Check sheet for the modelled part. Datum: model origin and axes. Units: mm. A direction names the side the tool comes from. Give positions to 0.01 mm unless a question says otherwise; leave off trailing zeros. Loops run counter-clockwise (first coordinate to the right, second up) from the corner with the lowest first, then second, coordinate; pieces in that order, holes last. Notation, with made-up numbers: (-7.75, 86) -> (20.25, 86) arc R11 cw to (20.25, 95) -> close; hole circle Ø8 at (72.25, 88.5). An arc over 180 degrees is marked (long way). Answer as CSV lines item,"result". Start each with the question number.
(1) Material ranges on line 1 (X direction, y = 23.4, z = 125); line 2 (Z direction, x = 0, y = 195); line 3 (X direction, y = 9, z = -62), recorded low to high. Write a range as from..to.
(2) Gauge pin test, flat ends, axial feed: pin 1 Ø19 at (x, y) = (0, 145) entering from -Z; pin 2 Ø13.5 at (y, z) = (108, 73) entering from -X; pin 3 Ø4 at (y, z) = (22, 116) entering from +X. Record the tip position at first contact, or that the pin passes through.
(3) Access from +Z, -Z, +X, -X, +Y, -Y to the whole of each face (thin tool, end or side, straight path). Record for faces 1 (the face through (-1.301, 150.857, 49.223)), 2 (the face through (-17.5, 131, 75)), 3 (the face through (97, 25, -56)), 4 (the face through (92.07, 22.46, -67.59)), 5 (the face through (106, 16.4, -45)).
(4) Release check for a two-part mould opening along Y. For faces 6 (the face through (-97, 25, -56)), 7 (the face through (2.956, 150.684, 73.907)), 8 (the face through (-47.69, 197.54, -15.02)) record: pulls with the +Y half, pulls with the -Y half, needs draft (parallel to the pull), parting line crosses it, or undercut.
(5) Section check A-A on z = 0. Enter the section's corners in (x, y), plus the area to 3 significant figures.
(6) Section check C-C on x = 0. State how many separate pieces and enclosed holes the cut face has, plus the area to 3 significant figures.
(7) Section check B-B on y = 97. Enter the section's corners in (x, z), plus the area to 3 significant figures.
from build123d import *

# Parameters (mm, degrees)
BOSS_EXTRUDE1_DEPTH = 80
HOLE1_D             = 50
HOLE1_CBORE_D       = 70
HOLE1_CBORE_DEPTH   = 12
BOSS_EXTRUDE2_DEPTH = 10
CIRPATTERN1_COUNT   = 3
FILLET1_R           = 5
HOLE2_D             = 13
HOLE2_CBORE_D       = 22
HOLE2_CBORE_DEPTH   = 5


with BuildPart() as part:
    # Sketch1 → Revolve1 (revolve)
    with BuildSketch(Plane.XY):
        Polygon((-150, 0), (-150, 15), (-106.265538433, 15), (-50, 195), (-50, 200), (0, 200), (0, 0), align=None)
    revolve(axis=Axis((0, 200, 0), (0, -1, 0)))

    # Sketch2 → Boss-Extrude1 (add)
    with BuildSketch(Plane.XY):
        with BuildLine():
            Line((-17.5, 145), (-17.5, 90))
            Line((-17.5, 90), (17.5, 90))
            Line((17.5, 90), (17.5, 145))
            ThreePointArc((17.5, 145), (0, 162.5), (-17.5, 145))
        make_face()
    extrude(amount=BOSS_EXTRUDE1_DEPTH)

    # Sketch4 → Cut-Revolve1 (revolve, cut)
    with BuildSketch(Plane(origin=(0, 0, 0), x_dir=(0, 0, -1), z_dir=(1, 0, 0)), mode=Mode.PRIVATE) as cut_revolve1_sk:
        Polygon((0, 151), (-73.5, 151), (-80, 157.5), (-80, 145), (0, 145), align=None)
    revolve(cut_revolve1_sk.sketch.rotate(Axis((0, 145, 80), (0, 0, -1)), 90), axis=Axis((0, 145, 80), (0, 0, -1)), mode=Mode.SUBTRACT)

    # Hole1 (through all)
    with Locations(Plane(origin=(0, 200, 0), x_dir=(1, 0, 0), z_dir=(0, 1, 0))):
        with Locations((0, 0)):
            CounterBoreHole(HOLE1_D / 2, HOLE1_CBORE_D / 2, HOLE1_CBORE_DEPTH)

    # Sketch7 → Cut-Revolve2 (revolve, cut)
    with BuildSketch(Plane(origin=(0, 0, 0), x_dir=(0, 0, -1), z_dir=(1, 0, 0)), mode=Mode.PRIVATE) as cut_revolve2_sk:
        with BuildLine():
            Line((0, 0), (90, 0))
            Line((90, 0), (53.93166414, 115.38680044))
            ThreePointArc((53.93166414, 115.38680044), (46.296011996, 121), (38.660359853, 115.38680044))
            Line((38.660359853, 115.38680044), (26.973757314, 78))
            Line((26.973757314, 78), (0, 78))
            Line((0, 78), (0, 0))
        make_face()
    revolve(cut_revolve2_sk.sketch.rotate(Axis((0, 78, 0), (0, -1, 0)), 180), axis=Axis((0, 78, 0), (0, -1, 0)), mode=Mode.SUBTRACT)

    # Sketch10 → Boss-Extrude2 (add)
    with BuildSketch(Plane(origin=(0, 15, 0), x_dir=(1, 0, 0), z_dir=(0, 1, 0))):
        with BuildLine():
            Line((-12.5, -125), (-12.5, -100))
            Line((-12.5, -100), (12.5, -100))
            Line((12.5, -100), (12.5, -125))
            ThreePointArc((12.5, -125), (0, -137.5), (-12.5, -125))
        make_face()
    boss_extrude2 = extrude(amount=BOSS_EXTRUDE2_DEPTH)

    # CirPattern1: Boss-Extrude2 ×3 about axis
    cirpattern1_axis = Axis((0, 0, 0), (0, 1, 0))
    for i in range(1, CIRPATTERN1_COUNT):
        add(boss_extrude2.rotate(cirpattern1_axis, i * 360 / CIRPATTERN1_COUNT))

    # Fillet1
    fillet1_edges = [part.edges().sort_by_distance(p)[0] for p in [
        (93.571461612, 15, -68.45726528),
        (119.07849302, 15, -68.75),
        (12.5, 15, 115.263895465),
        (0, 15, 137.5),
        (-93.571461612, 15, -68.45726528),
        (-119.07849302, 15, -68.75),
        (106.071461612, 15, -46.806630185),
        (-12.5, 15, 115.263895465),
        (-106.071461612, 15, -46.806630185),
    ]]
    fillet(fillet1_edges, radius=FILLET1_R)

    # Hole2 (through all)
    with Locations(Plane(origin=(0, 25, 0), x_dir=(1, 0, 0), z_dir=(0, 1, 0))):
        with Locations((108.253175473, 62.5), (-108.253175473, 62.5), (0, -125)):
            CounterBoreHole(HOLE2_D / 2, HOLE2_CBORE_D / 2, HOLE2_CBORE_DEPTH)


solid = part.part
Working result:
1,line 1,"x = -12.5..-11, 11..12.5"
1,line 2,"z = -50..-35, 35..50"
1,line 3,"x = -136.59..-114.73, -101.77..-61.3, 61.3..101.77, 114.73..136.59"
2,pin 1,"stops at z = -68.6"
2,pin 2,"stops at x = -40.35"
2,pin 3,"stops at x = 12.5"
3,face 1,"+Z"
3,face 2,"+Z, -X, +Y"
3,face 3,"-Z, +X, +Y"
3,face 4,"-Z, +Y"
3,face 5,"+X, +Y"
4,face 6,"pulls with the +Y half"
4,face 7,"undercut"
4,face 8,"needs draft"
5,outline,"(-150, 0) -> (-90, 0) -> (-53.93, 115.39) arc R8 cw to (-38.66, 115.39) -> (-26.97, 78) -> (-25, 78) -> (-25, 188) -> (-35, 188) -> (-35, 200) -> (-50, 200) -> (-50, 195) -> (-106.27, 15) -> (-150, 15) -> close; (25, 78) -> (26.97, 78) -> (38.66, 115.39) arc R8 cw to (53.93, 115.39) -> (90, 0) -> (150, 0) -> (150, 15) -> (106.27, 15) -> (50, 195) -> (50, 200) -> (35, 200) -> (35, 188) -> (25, 188) -> close"
5,area,"12,500 mm^2"
6,separate pieces,"4"
6,enclosed holes,"0"
6,area,"12,400 mm^2"
7,outline,"circle Ø65.83 at (0, 0); (-17.5, 78.71) arc R80.63 ccw (long way) to (17.5, 78.71) -> (17.5, 80) -> (10.09, 80) arc R80.63 ccw to (-10.09, 80) -> (-17.5, 80) -> close; hole circle Ø119.36 at (0, 0); hole circle Ø50 at (0, 0)"
7,area,"10,700 mm^2"
